Part model, mm, in its own coordinate system. A direction names the side the tool comes from. Coordinates: 2 decimals unless noted, no trailing zeros. Loops run counter-clockwise (first coordinate to the right, second up) from the corner with the lowest first, then second, coordinate; pieces in that order, holes last. Notation, with made-up numbers: (45.25, 20) - (103.25, 20) arc R10 ccw to (103.25, 27) - close; hole circle Ø9 at (65.25, 35). An arc over 180 degrees is marked (long way). Use a Markdown table: item, result. Add a question column.
1. Wall check: probe 1 along Z at (x, y) = (-2.25, 1.75); probe 2 along X at (y, z) = (0.25, 4.1); probe 3 along Z at (x, y) = (3.5, 2.5). Give the ranges that are in metal, low to high. Write a range as [from, to].
2. 3-axis set-ups, long thin cutter, end or side, ignore diameter. For faces 1 (the cylindrical face through (-0.59, -4.46, 3.06)), 2 (the cylindrical face through (-0.338, -2.578, 0.989)): which of +Z, -Z, +X, -X, +Y, -Y reach the whole face in a straight line?
3. Band-saw the part on C-C, the plane z = 2.85. Give the cut face in (x, y).
4. Drop flat-ended pins along their axis: pin 1 (1.5 mm diameter, centred on y = -2, z = 4.5, fed in from -X); pin 2 (2 mm diameter, centred on y = 3, z = 3, fed in from +X). Give the stop position or say it passes through.
5. Band-saw the part on D-D, the plane z = 1.35. Give the cut face in (x, y).
from build123d import *

# Parameters (mm, degrees)
F2_SIZE = 1
F3_SIZE = 0.24999


# Not quite as in the source:
# - a fillet or chamfer is up to 0.001 mm smaller than in the source, because OpenCascade refuses the exact size


with BuildPart() as f1:
    # F0 (on Front) → F1 (revolve)
    with BuildSketch(Plane.XZ):
        Polygon((0, 4.8), (0, 0), (2.6, 0), (2.6, 2.2), (2.35, 2.2), (2.35, 2.3), (2.6, 2.3), (4.5, 2.3), (4.5, 4.8), align=None)
    revolve(axis=Axis((0, 0, 2.4), (0, 0, -1)))

    # F2
    f2_edges = [f1.edges().sort_by_distance(p)[0] for p in [
        (-4.5, 0, 4.8),
    ]]
    chamfer(f2_edges, length=F2_SIZE)

    # F3 (size 0.25 in the source; OpenCascade refuses exactly that, so slightly less here)
    f3_edges = [f1.edges().sort_by_distance(p)[0] for p in [
        (-2.6, 0, 2.2),
    ]]
    chamfer(f3_edges, length=F3_SIZE)


solid = f1.part
Geometry check:
| question | item | result |
|---|---|---|
| 1 | probe 1 | z = [2.3, 4.8] |
| 1 | probe 2 | x = [-4.19, 4.19] |
| 1 | probe 3 | z = [2.3, 4] |
| 2 | face 1 | +Z, -Z |
| 2 | face 2 | -Z |
| 3 | outline | circle Ø9 at (0, 0) |
| 4 | pin 1 | stops at x = -4.15 |
| 4 | pin 2 | stops at x = 4.03 |
| 5 | outline | circle Ø5.2 at (0, 0) |
